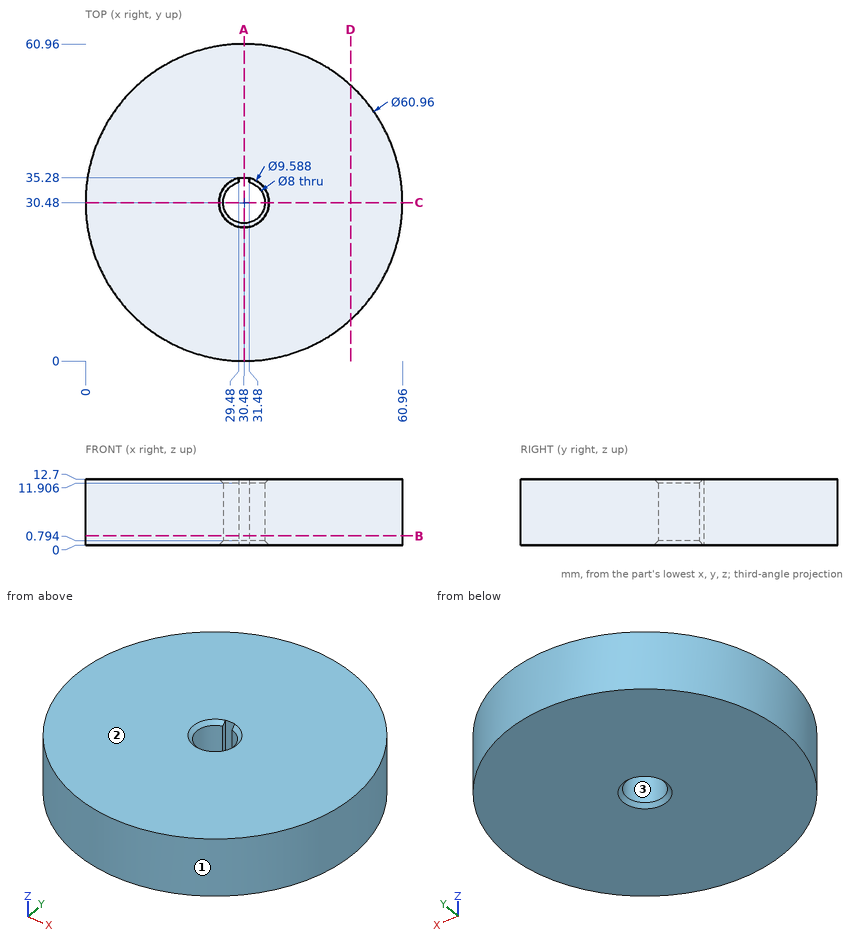
Source: three-view drawing plus pictorial views. Frame: mm from the lowest corner of the part. Round coordinates to 2 decimals unless told otherwise and drop trailing zeros. Loops run counter-clockwise (first coordinate to the right, second up) from the corner with the lowest first, then second, coordinate; pieces in that order, holes last. Notation, with made-up numbers: (-23, 53.5) -> (5, 53.5) arc R19 ccw to (5, 70.5) -> close; hole circle Ø3 at (49, 23.5). An arc over 180 degrees is marked (long way). Use one line per item in the form item = value.
Item 1: Cut plane D-D on x = 51. Output: boundary loops of the cut face in (y, z).
Evaluation:
outline = (7.94, 0) -> (53.02, 0) -> (53.02, 12.7) -> (7.94, 12.7) -> close
Item 2: Cut plane B-B on z = 1.75. Output: boundary loops of the cut face in (x, y).
Evaluation:
outline = circle Ø60.96 at (30.48, 30.48); hole (29.48, 34.35) arc R4 ccw (long way) to (31.48, 34.35) -> (31.48, 35.28) -> (29.48, 35.28) -> close
Item 3: Material intervals for probe 1 along Y at (x, z) = (30.48, 5.5); probe 2 along X at (y, z) = (34, 3.75) (1 decimal); probe 3 along Y at (x, z) = (5.5, 10) (1 decimal), sorted ascending.
Evaluation:
probe_1 = 0 to 26.48, 35.28 to 60.96
probe_2 = 0.2 to 28.6, 32.4 to 60.8
probe_3 = 13 to 47.9
Item 4: Cut plane A-A on x = 30.48. Output: boundary loops of the cut face in (y, z), then the cut area to 3 significant figures.
Evaluation:
outline = (0, 0) -> (25.69, 0) -> (26.48, 0.79) -> (26.48, 11.91) -> (25.69, 12.7) -> (0, 12.7) -> close; (35.28, 0) -> (60.96, 0) -> (60.96, 12.7) -> (35.28, 12.7) -> close
area = 662 mm2
Item 5: Contact query for flat-ended pins moving along their axis: pin 1 Ø0.5 at (y, z) = (35, 3.5) entering from +X; pin 2 Ø9 at (x, y) = (30.48, 30.48) entering from +Z (1 decimal); pin 3 Ø5 at (x, z) = (51, 6) entering from +Y. Output: stop coordinate, or through.
Evaluation:
pin_1 = 60.66
pin_2 = 12.4
pin_3 = 55.06
Item 6: Cut plane C-C on y = 30.48. Output: boundary loops of the cut face in (x, z).
Evaluation:
outline = (0, 0) -> (25.69, 0) -> (26.48, 0.79) -> (26.48, 11.91) -> (25.69, 12.7) -> (0, 12.7) -> close; (34.48, 0.79) -> (35.27, 0) -> (60.96, 0) -> (60.96, 12.7) -> (35.27, 12.7) -> (34.48, 11.91) -> close
Item 7: Draft query along X for the marked faces 1, 2 and 3. Return one class per face: released by +X, released by -X, zero draft, split by the parting line, or undercut.
Evaluation:
face_1 = split by the parting line
face_2 = zero draft
face_3 = undercut
